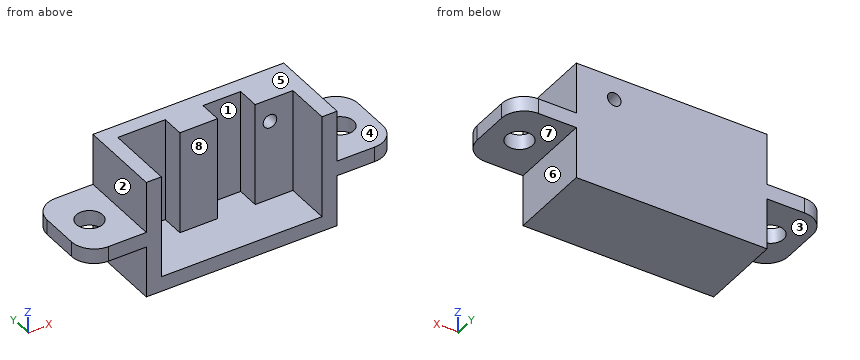
from build123d import *

# Parameters (mm, degrees)
F0_W      = 25.32
F0_H      = 15.7
F1_DEPTH  = 2
F3_DEPTH  = 9
F4_W      = 5
F4_H      = 13.7
F5_DEPTH  = 3
F6_R      = 0.9
F7_DEPTH  = 5.001
F8_W      = 11
F8_H      = 2
F9_DEPTH  = 8
F10_R     = 3
F11_W     = 11
F11_H     = 2
F12_DEPTH = 8
F13_R     = 3
F14_R     = 1.75
F15_DEPTH = 8.851
F16_R     = 1.75
F17_DEPTH = 8.851


with BuildPart() as f1:
    # F0 (on Front) → F1 (new body)
    with BuildSketch(Plane.XZ):
        with Locations((10.16, 5.35)):
            Rectangle(F0_W, F0_H)
    extrude(amount=F1_DEPTH)

    # F2 (on face) → F3 (join)
    with BuildSketch(Plane.XZ.offset(2)):
        Polygon((-2.5, 13.2), (-2.5, -2.5), (22.82, -2.5), (22.82, 13.2), (20.82, 13.2), (20.82, -0.5), (-0.5, -0.5), (-0.5, 13.2), align=None)
    extrude(amount=F3_DEPTH)

    # F4 (on face) → F5 (join)
    with BuildSketch(Plane.XZ.offset(2)):
        with Locations((8.32, 6.35)):
            Rectangle(F4_W, F4_H)
        with Locations((18.32, 6.35)):
            Rectangle(F4_W, F4_H)
    extrude(amount=F5_DEPTH)

    # F6 (on face) → F7 (cut, through all)
    with BuildSketch(Plane.XZ.offset(5)):
        with Locations((17.78, 10.16)):
            Circle(F6_R)
    extrude(amount=-F7_DEPTH, mode=Mode.SUBTRACT)

    # F8 (on face) → F9 (join)
    with BuildSketch(Plane(origin=(-2.5, 0, 0), x_dir=(0, -1, 0), z_dir=(-1, 0, 0))):
        with Locations((5.5, 5.35)):
            Rectangle(F8_W, F8_H)
    extrude(amount=F9_DEPTH)

    # F10
    f10_edges = [f1.edges().sort_by_distance(p)[0] for p in [
        (-10.5, -11, 5.35),
        (-10.5, 0, 5.35),
    ]]
    fillet(f10_edges, radius=F10_R)

    # F11 (on face) → F12 (join)
    with BuildSketch(Plane.YZ.offset(22.82)):
        with Locations((-5.5, 5.35)):
            Rectangle(F11_W, F11_H)
    extrude(amount=F12_DEPTH)

    # F13
    f13_edges = [f1.edges().sort_by_distance(p)[0] for p in [
        (30.82, -11, 5.35),
        (30.82, 0, 5.35),
    ]]
    fillet(f13_edges, radius=F13_R)

    # F14 (on face) → F15 (cut, through all)
    with BuildSketch(Plane.XY.offset(6.35)):
        with Locations((-6.5, -5.5)):
            Circle(F14_R)
    extrude(amount=-F15_DEPTH, mode=Mode.SUBTRACT)

    # F16 (on face) → F17 (cut, through all)
    with BuildSketch(Plane.XY.offset(6.35)):
        with Locations((26.82, -5.5)):
            Circle(F16_R)
    extrude(amount=-F17_DEPTH, mode=Mode.SUBTRACT)


solid = f1.part
For this review, take the finished solid that the model builds, in its own axes (mm). Face numbers are marked on the shaded views. A direction names the side the tool comes from. Coordinates: 2 decimals unless noted, no trailing zeros. Loops run counter-clockwise (first coordinate to the right, second up) from the corner with the lowest first, then second, coordinate; pieces in that order, holes last. Notation, with made-up numbers: (72.5, 20.25) - (120.5, 20.25) arc R20 ccw to (120.5, 53.25) - close; hole circle Ø3 at (-22.5, 69). An arc over 180 degrees is marked (long way). Return JSON: item names as keys, results as strings.
Item 1: For the marked faces 1, 2, 3, 4 and 5, list the 3-axis set-ups (+Z, -Z, +X, -X, +Y, -Y) from which the entire face can be reached by the end or side of a thin tool; tool diameter is ignored.
Determined:
{"face 1": "+Z, -Y", "face 2": "+Z, -X, +Y, -Y", "face 3": "-Z, -X, +Y, -Y", "face 4": "+Z, +X, +Y, -Y", "face 5": "+Z, +X, -X, +Y, -Y"}
Item 2: Take a section at C-C (y = -5.5). Give the boundary of the cut face in (x, z).
Determined:
{"outline": "(-10.5, 4.35) - (-8.25, 4.35) - (-8.25, 6.35) - (-10.5, 6.35) - close; (-4.75, 4.35) - (-2.5, 4.35) - (-2.5, -2.5) - (22.82, -2.5) - (22.82, 4.35) - (25.07, 4.35) - (25.07, 6.35) - (22.82, 6.35) - (22.82, 13.2) - (20.82, 13.2) - (20.82, -0.5) - (-0.5, -0.5) - (-0.5, 13.2) - (-2.5, 13.2) - (-2.5, 6.35) - (-4.75, 6.35) - close; (28.57, 4.35) - (30.82, 4.35) - (30.82, 6.35) - (28.57, 6.35) - close"}
Item 3: Take a section at B-B (z = 10.16). Give the boundary of the cut face in (x, y).
Determined:
{"outline": "(-2.5, -11) - (-0.5, -11) - (-0.5, -2) - (5.82, -2) - (5.82, -5) - (10.82, -5) - (10.82, -2) - (15.82, -2) - (15.82, -5) - (16.88, -5) - (16.88, 0) - (-2.5, 0) - close; (18.68, -5) - (20.82, -5) - (20.82, -11) - (22.82, -11) - (22.82, 0) - (18.68, 0) - close"}
Item 4: Insertion check: pin 1 (1.5 mm diameter, centred on x = 15, z = 3, fed in from -Y); pin 2 (5.5 mm diameter, centred on y = -6, z = -0.5, fed in from +X); pin 3 (2.5 mm diameter, centred on x = 12, z = 7.5, fed in from -Y). Each pin has a flat end and moves straight along its axis. Give the tip position at first contact, or say it passes through.
Determined:
{"pin 1": "stops at y = -2", "pin 2": "stops at x = 22.82", "pin 3": "stops at y = -5"}
Item 5: Take a section at D-D (z = 1.5). Give the boundary of the cut face in (x, y), then the cut area to 3 significant figures.
Determined:
{"outline": "(-2.5, -11) - (-0.5, -11) - (-0.5, -2) - (5.82, -2) - (5.82, -5) - (10.82, -5) - (10.82, -2) - (15.82, -2) - (15.82, -5) - (20.82, -5) - (20.82, -11) - (22.82, -11) - (22.82, 0) - (-2.5, 0) - close", "area": "117 mm2"}
Item 6: Mouldability with a two-part tool opening along X and no side actions: class the marked faces 6, 7 and 8 as pulls with the +X half, pulls with the -X half, needs draft (parallel to the pull), parting line crosses it, or undercut.
Determined:
{"face 6": "pulls with the +X half", "face 7": "needs draft", "face 8": "undercut"}
Item 7: Take a section at A-A (x = 17.78). Give the boundary of the cut face in (y, z), then the cut area to 3 significant figures.
Determined:
{"outline": "(-11, -2.5) - (0, -2.5) - (0, 9.26) - (-5, 9.26) - (-5, -0.5) - (-11, -0.5) - close; (-5, 11.06) - (0, 11.06) - (0, 13.2) - (-5, 13.2) - close", "area": "81.5 mm2"}
Item 8: For line 1 (X direction, y = -8.75, z = 3.5); line 2 (X direction, y = -3, z = 0); line 3 (Y direction, x = 26.82, z = 5.85), list the stretches that pass through material, from the lowest coordinate up.
Determined:
{"line 1": "x = -2.5 to -0.5, 20.82 to 22.82", "line 2": "x = -2.5 to -0.5, 5.82 to 10.82, 15.82 to 22.82", "line 3": "y = -11 to -7.25, -3.75 to 0"}
